Autodesk Inventor part; units mm, degrees
ref_plane "YZ Plane" through (0, 0, 0) normal (1, 0, 0) x (0, 1, 0)
ref_plane "XZ Plane" through (0, 0, 0) normal (0, 1, 0) x (-1, 0, 0)
ref_plane "XY Plane" through (0, 0, 0) normal (0, 0, 1) x (1, 0, 0)
sketch "Skizze1" plane through (0, 0, 0) normal (0, 0, 1) x (1, 0, 0)
  line L0 (0, 0) -> (-13, 0)
  line L1 (-13, 0) -> (-13, -0.46)
  line L2 (-13, -0.46) -> (-10, -0.46)
  line L3 (-10, -0.46) -> (-10, -3.62)
  line L4 (-10, -3.62) -> (-13, -3.62)
  line L5 (-13, -3.62) -> (-13, -4.08)
  line L6 (-13, -4.08) -> (0, -4.08)
  line L7 (0, -4.08) -> (0, 0)
  line L8 (0, -4.825) -> (-13, -4.825)
  line L9 (-13, -4.825) -> (-13, -5.285)
  line L10 (-13, -5.285) -> (-10, -5.285)
  line L11 (-10, -5.285) -> (-10, -8.445)
  line L12 (-10, -8.445) -> (-13, -8.445)
  line L13 (-13, -8.445) -> (-13, -8.905)
  line L14 (-13, -8.905) -> (0, -8.905)
  line L15 (0, -8.905) -> (0, -4.825)
  dimension "d0" = 13
  dimension "d1" = 0.46
  dimension "d2" = 3
  dimension "d3" = 3.16
  dimension "d4" = 0.46
  dimension "d7" = 4.825
revolve "Umdrehung1" add sketch "Skizze1" angle 360 about axis through (0, -8.905, 0) along (0, 1, 0)
sketch "Skizze2" plane through (0, 0, 0) normal (0, 1, 0) x (1, 0, 0)
  line L0 (6.25, -14.6) -> (-6.25, -14.6)
  line L1 (-6.25, -14.6) -> (-6.25, -5.3061)
  line L2 (-6.25, -5.3061) -> (6.25, -5.3061)
  line L3 (6.25, -5.3061) -> (6.25, -14.6)
  line L4 (6.25, -14.6) -> (-6.25, -5.3061) construction
  line L5 (-6.25, -14.6) -> (6.25, -5.3061) construction
  point P0 (0, 0)
  point P1 (0, -9.9531)
  dimension "d13" = 12.5
  dimension "d14" = 14.6
extrude "Extrusion1" add sketch "Skizze2" along normal blind 7.4 and the other way blind 7
sketch "Skizze3" plane through (0, -8.905, 0) normal (0, -1, 0) x (1, 0, 0)
  circle A0 centre (0, 0) radius 13
  circle A1 centre (0, 0) radius 6
  dimension "d19" = 12
extrude "Extrusion2" cut sketch "Skizze3" against normal through all contours A1
properties part number "50_ETL_28by_coil"
The model under review builds one solid part; all positions refer to its coordinate system, in mm. A direction names the side the tool comes from. Round coordinates to 2 decimals unless told otherwise and drop trailing zeros. Loops run counter-clockwise (first coordinate to the right, second up) from the corner with the lowest first, then second, coordinate; pieces in that order, holes last. Notation, with made-up numbers: M 51,-22 L 108,-22 A5 ccw 108,-14 Z; hole C -5.5,73 d8. An arc over 180 degrees is marked long. Write item = value, one per line.
Item 1: Take a section at B-B on x = 0. Write out the cut boundary in (y, z) (3 decimals).
Return value:
outline = M -8.905,-13 L -8.445,-13 L -8.445,-10 L -5.285,-10 L -5.285,-13 L -4.825,-13 L -4.825,-6 L -8.905,-6 Z; M -8.905,6 L 7.4,6 L 7.4,14.6 L -7,14.6 L -7,10 L -8.445,10 L -8.445,13 L -8.905,13 Z; M -4.08,-13 L -3.62,-13 L -3.62,-10 L -0.46,-10 L -0.46,-13 L 0,-13 L 0,-6 L -4.08,-6 Z
Item 2: Take a section at D-D on x = -11.25. Write out the cut boundary in (y, z) (3 decimals).
Return value:
outline = M -8.905,-6.514 L -8.445,-6.514 L -8.445,6.514 L -8.905,6.514 Z; M -5.285,-6.514 L -4.825,-6.514 L -4.825,6.514 L -5.285,6.514 Z; M -4.08,-6.514 L -3.62,-6.514 L -3.62,6.514 L -4.08,6.514 Z; M -0.46,-6.514 L 0,-6.514 L 0,6.514 L -0.46,6.514 Z
Item 3: Machinability: for faces 4 (the cylindrical face through (10.316, -8.678, 7.91)), 5 (the flat face through (-7, -8.445, -8)), 6 (the flat face through (-6.25, 2, 10)), 7 (the flat face through (-5, 4, 5.306)), which of the approach directions +Z, -Z, +X, -X, +Y, -Y give a long, thin tool a straight path to every point of the face, cutting with its end or side? Answer none if there is none.
Return value:
face_4 = -Y
face_5 = none
face_6 = +Z, -X
face_7 = -Z, +X, -X, +Y
Item 4: Insertion check: P1, Ø1, axis at y = -7, z = -6.5, coming from the -X side; P2, Ø4, axis at x = -4, y = 4, coming from the -Z side; P3, Ø7.5, axis at x = -2.5, z = -4.5, coming from the +Y side. Each pin has a flat end and moves straight along its axis. Give the tip position at first contact, or say it passes through.
Return value:
P1 = -8
P2 = 5.31
P3 = 0
Item 5: Take a section at C-C on y = 5.5. Write out the cut boundary in (x, z), then the cut area to 3 significant figures.
Return value:
outline = M -6.25,5.31 L -2.8,5.31 A6 cw 2.8,5.31 L 6.25,5.31 L 6.25,14.6 L -6.25,14.6 Z
area = 114 mm2
Item 6: For line 1 (Y direction, x = 7, z = 8.25) (3 decimals); line 2 (Y direction, x = 7.75, z = 3.25) (3 decimals); line 3 (X direction, y = -1.5, z = 0), list the stretches that pass through material, from the lowest coordinate up. Write a range as [from, to].
Return value:
line_1 = [-8.905, -8.445], [-5.285, -4.825], [-4.08, -3.62], [-0.46, 0]
line_2 = [-8.905, -4.825], [-4.08, 0]
line_3 = [-10, -6], [6, 10]
Item 7: Take a section at A-A on z = 0. State how many separate pieces and enclosed holes the cut face has, then the cut area to 3 significant figures.
Return value:
separate_pieces = 4
enclosed_holes = 0
area = 76.3 mm2
Item 8: The part is to be moulded in two halves that separate along Y. For faces 1 (the flat face through (6.25, 2, 10)), 2 (the cylindrical face through (0, -5, -13)), 3 (the flat face through (-6, -8.905, -3)), say which applies: released by +Y, released by -Y, zero draft, split by the parting line, or undercut.
Return value:
face_1 = undercut
face_2 = zero draft
face_3 = released by -Y
